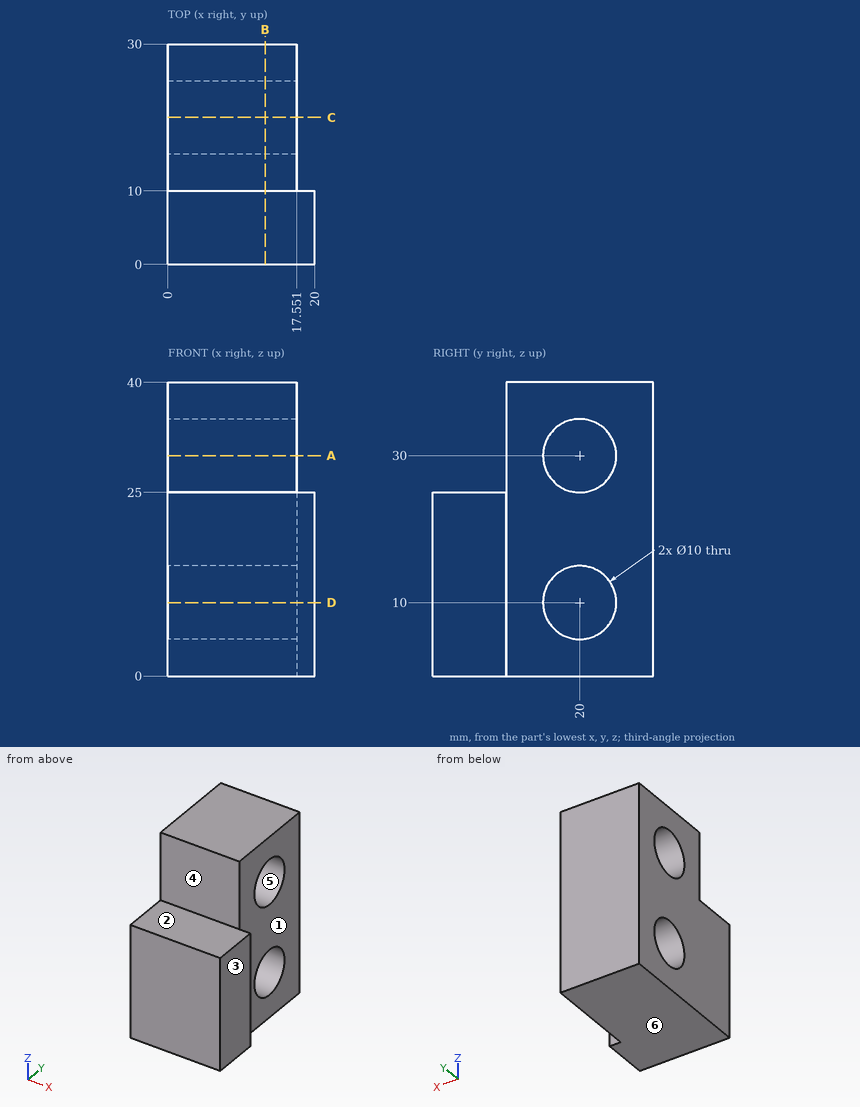
Can you work these out from the drawing? Everything is in mm from the part's minimum corner. A direction names the side the tool comes from. Give positions to 0.01 mm unless a question says otherwise; leave off trailing zeros. Order: outer loops, then holes, each group sorted by start corner. A loop starts at its lowest first (then second) coordinate and runs counter-clockwise, first axis right, second up. Notation, with made-up numbers: (38.25, 45.25) -> (62.25, 45.25) arc R31 ccw to (62.25, 77.25) -> close; hole circle Ø10 at (20, 83.5). An arc over 180 degrees is marked (long way). Return JSON: item names as keys, results as strings.
1. For pin 1 Ø11.5 at (y, z) = (20, 10) entering from +X; pin 2 Ø1.2 at (x, z) = (18.5, 14.5) entering from +Y; pin 3 Ø4.5 at (x, z) = (12, 34) entering from -Y; pin 4 Ø9 at (y, z) = (20, 30) entering from -X, each with a flat end and sliding along its axis, tell me the tip position at first contact or that it passes through.
Answer list:
{"pin 1": "stops at x = 17.55", "pin 2": "stops at y = 10", "pin 3": "stops at y = 10", "pin 4": "passes through"}
2. Thinking about a two-plate mould opening in Y: for the marked faces 4, 5 and 6, which applies, pulls with the +Y half, pulls with the -Y half, needs draft (parallel to the pull), parting line crosses it, or undercut?
Answer list:
{"face 4": "pulls with the -Y half", "face 5": "undercut", "face 6": "needs draft"}
3. Imagine slicing it at A-A on z = 30. List the corners of the cut face in (x, y) for me.
Answer list:
{"outline": "(0, 10) -> (17.55, 10) -> (17.55, 15) -> (0, 15) -> close; (0, 25) -> (17.55, 25) -> (17.55, 30) -> (0, 30) -> close"}
4. Imagine slicing it at B-B on x = 13.25. List the corners of the cut face in (y, z) for me.
Answer list:
{"outline": "(0, 0) -> (30, 0) -> (30, 40) -> (10, 40) -> (10, 25) -> (0, 25) -> close; hole circle Ø10 at (20, 10); hole circle Ø10 at (20, 30)"}
5. Imagine slicing it at D-D on z = 10. List the corners of the cut face in (x, y) for me.
Answer list:
{"outline": "(0, 0) -> (20, 0) -> (20, 10) -> (17.55, 10) -> (17.55, 15) -> (0, 15) -> close; (0, 25) -> (17.55, 25) -> (17.55, 30) -> (0, 30) -> close"}
6. On a 3-axis mill with a long thin cutter (end or side, diameter ignored), from which of +Z, -Z, +X, -X, +Y, -Y can I reach the whole of each face in a straight line? I mean the marked faces 1, 2 and 3. Say none if no direction works.
Answer list:
{"face 1": "+Z, -Z, +X, +Y", "face 2": "+Z, +X, -X, -Y", "face 3": "+Z, -Z, +X, +Y, -Y"}
7. Imagine slicing it at C-C on y = 20. List the corners of the cut face in (x, z) for me.
Answer list:
{"outline": "(0, 0) -> (17.55, 0) -> (17.55, 5) -> (0, 5) -> close; (0, 15) -> (17.55, 15) -> (17.55, 25) -> (0, 25) -> close; (0, 35) -> (17.55, 35) -> (17.55, 40) -> (0, 40) -> close"}
8. I need wall thicknesses on line 1 (Z direction, x = 5.25, y = 20); line 2 (Y direction, x = 18.5, z = 9); line 3 (Y direction, x = 10.5, z = 30.5) (1 decimal). Which ranges of each line are inside material? Lowest first, please. Write a range as from..to.
Answer list:
{"line 1": "z = 0..5, 15..25, 35..40", "line 2": "y = 0..10", "line 3": "y = 10..15, 25..30"}
